Source: CAD feature listing. Evaluate the final solid. Frame: model axes, mm. Face numbers are marked on the shaded views. Give positions to 0.01 mm unless a question says otherwise; leave off trailing zeros. Order: outer loops, then holes, each group sorted by start corner. A loop starts at its lowest first (then second) coordinate and runs counter-clockwise, first axis right, second up.
```python
from build123d import *

# Parameters (mm, degrees)
SKETCH002_W            = 65
SKETCH002_H            = 110
SKETCH002_W_2          = 61
SKETCH002_H_2          = 106
PAD002_DEPTH           = 5
SKETCH003_W            = 65
SKETCH003_H            = 110
SKETCH003_W_2          = 23.5
SKETCH003_H_2          = 98.676263
SKETCH003_H_3          = 24.954477
SKETCH003_H_4          = 22.149553
SKETCH003_H_5          = 22.384941
SKETCH003_H_6          = 10.511029
PAD003_DEPTH           = 2
PAD001_DEPTH           = 10
SKETCH_W               = 59
SKETCH_H               = 10
PAD_DEPTH              = 2
FUSION_PLACEMENT_ANGLE = -33.7
FILLET_R               = 1
FILLET001_R            = 4
FILLET002_R            = 4
FILLET003_R            = 2


with BuildPart() as pad002:
    # Sketch002 → Pad002 (new body)
    with BuildSketch(Plane.XY):
        with Locations((32.5, -56.5)):
            Rectangle(SKETCH002_W, SKETCH002_H)
        with Locations((32.5, -56.5)):
            Rectangle(SKETCH002_W_2, SKETCH002_H_2, mode=Mode.SUBTRACT)
    extrude(amount=PAD002_DEPTH)


with BuildPart() as fusion001:
    # Sketch003 → Pad003 (new body)
    with BuildSketch(Plane.XY):
        with Locations((32.5, -56.5)):
            Rectangle(SKETCH003_W, SKETCH003_H)
        with Locations((17.75, -56.838131)):
            Rectangle(SKETCH003_W_2, SKETCH003_H_2, mode=Mode.SUBTRACT)
        with Locations((47.25, -19.977238)):
            Rectangle(SKETCH003_W_2, SKETCH003_H_3, mode=Mode.SUBTRACT)
        with Locations((47.25, -49.529253)):
            Rectangle(SKETCH003_W_2, SKETCH003_H_4, mode=Mode.SUBTRACT)
        with Locations((47.25, -77.7965)):
            Rectangle(SKETCH003_W_2, SKETCH003_H_5, mode=Mode.SUBTRACT)
        with Locations((47.25, -100.244485)):
            Rectangle(SKETCH003_W_2, SKETCH003_H_6, mode=Mode.SUBTRACT)
    extrude(amount=PAD003_DEPTH)

    # Fusion001: union Pad002
    add(pad002.part)


with BuildPart() as pad001:
    # Sketch001 → Pad001 (new body)
    with BuildSketch(Plane.XY):
        Polygon((0, 0), (0, -8.6), (2.6, -8.6), (2.6, -7.5), (1.1, -7.5), (1.1, -5.5), (2.6, -5.5), (2.6, -1.5), (56.4, -1.5), (56.4, -5.5), (57.9, -5.5), (57.9, -7.5), (56.4, -7.5), (56.4, -8.6), (59, -8.6), (59, 0), align=None)
    extrude(amount=PAD001_DEPTH)


with BuildPart() as relay001:
    # Sketch → Pad (new body)
    with BuildSketch(Plane.XY):
        with Locations((29.5, -5)):
            Rectangle(SKETCH_W, SKETCH_H)
    extrude(amount=PAD_DEPTH)

    # Fusion: union Pad001
    add(pad001.part)


with BuildPart() as relay001_1:
    # Fusion placement: moved
    add(relay001.part.moved(Location((5.548444, -1.680459, 0))).rotate(Axis((5.548444, -1.680459, 0), (0, 0, 1)), FUSION_PLACEMENT_ANGLE))


with BuildPart() as clone_of_relay002:
    # Clone001 base: copy of Relay001
    add(relay001_1.part)


with BuildPart() as clone_of_relay002_1:
    # Clone001 placement: moved
    add(clone_of_relay002.part.moved(Location((0, -56, 0))))


with BuildPart() as fillet003:
    # Clone base: copy of Relay001
    add(relay001_1.part)


with BuildPart() as fillet003_1:
    # Clone placement: moved
    add(fillet003.part.moved(Location((0, -28, 0))))

    # Fusion002: union Fusion001, Clone of Relay002, Relay001
    add(fusion001.part)
    add(clone_of_relay002_1.part)
    add(relay001_1.part)

    # Fillet
    fillet_edges = [fillet003_1.edges().sort_by_distance(p)[0] for p in [
        (49.085293, -98.735821, 1),
        (49.085293, -70.735821, 1),
        (49.085293, -42.735821, 1),
    ]]
    fillet(fillet_edges, radius=FILLET_R)

    # Fillet001
    fillet001_edges = [fillet003_1.edges().sort_by_distance(p)[0] for p in [
        (35.5, -94.988971, 1),
        (43.467128, -94.988971, 1),
        (51.584132, -94.988971, 1),
        (35.5, -66.60403, 1),
        (42.889933, -66.60403, 1),
        (51.840855, -66.60403, 1),
        (35.5, -38.454477, 1),
        (42.665688, -38.454477, 1),
        (51.940595, -38.454477, 1),
        (35.5, -7.5, 1),
        (35.5, -21.655663, 1),
        (51.692138, -32.454477, 1),
        (35.5, -49.655663, 1),
        (51.916383, -60.60403, 1),
        (35.5, -77.655663, 1),
        (52.493578, -88.988971, 1),
        (35.5, -105.5, 1),
        (59, -66.60403, 1),
        (59, -38.454477, 1),
        (59, -7.5, 1),
        (59, -94.988971, 1),
        (59, -105.5, 1),
        (59, -88.988971, 1),
        (59, -60.60403, 1),
        (59, -32.454477, 1),
    ]]
    fillet(fillet001_edges, radius=FILLET001_R)

    # Fillet002
    fillet002_edges = [fillet003_1.edges().sort_by_distance(p)[0] for p in [
        (29.5, -85.674054, 1),
        (29.5, -57.674054, 1),
        (29.5, -29.674054, 1),
        (6, -70.001503, 1),
        (6, -42.001503, 1),
        (6, -14.001503, 1),
        (6, -29.981609, 1),
        (6, -57.981609, 1),
        (6, -106.176263, 1),
        (29.5, -45.654161, 1),
        (29.5, -73.654161, 1),
        (29.5, -106.176263, 1),
    ]]
    fillet(fillet002_edges, radius=FILLET002_R)

    # Fillet003
    fillet003_edges = [fillet003_1.edges().sort_by_distance(p)[0] for p in [
        (29.5, -7.5, 1),
        (14.274478, -7.5, 1),
        (29.5, -17.654161, 1),
    ]]
    fillet(fillet003_edges, radius=FILLET003_R)


solid = fillet003_1.part
```
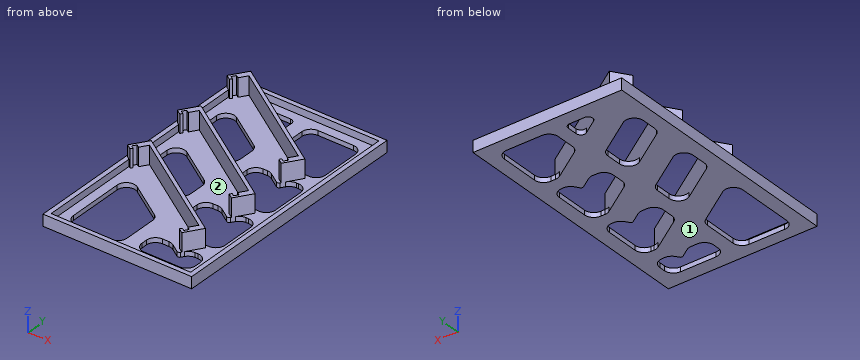
1) Draft query along X for the marked faces 1 and 2. Return one class per face: +X half, -X half, draft (parallel to the pull), parting line (faces both ways), or undercut.
Report:
face 1: draft
face 2: undercut
2) Section query C-C, the plane y = -26. Return the cut outline in (x, z).
Report:
outline: (0, 0) - (6, 0) - (6, 2) - (2, 2) - (2, 5) - (0, 5) - close; (23.99, 0) - (42.01, 0) - (42.01, 10) - (39.31, 10) - (39.31, 2) - (23.99, 2) - close; (59, 0) - (65, 0) - (65, 5) - (63, 5) - (63, 2) - (59, 2) - close
3) Section query B-B, the plane x = 15.5. Return the cut outline in (y, z).
Report:
outline: (-111.5, 0) - (-106.18, 0) - (-106.18, 2) - (-109.5, 2) - (-109.5, 5) - (-111.5, 5) - close; (-76.34, 0) - (-64.32, 0) - (-64.32, 10) - (-66.12, 10) - (-66.12, 2) - (-76.34, 2) - close; (-48.34, 0) - (-36.32, 0) - (-36.32, 10) - (-38.12, 10) - (-38.12, 2) - (-48.34, 2) - close; (-20.34, 0) - (-1.5, 0) - (-1.5, 5) - (-3.5, 5) - (-3.5, 2) - (-8.32, 2) - (-8.32, 10) - (-10.12, 10) - (-10.12, 2) - (-20.34, 2) - close
4) Section query D-D, the plane x = 33. Return the cut outline in (y, z), and give its area (3 significant figures).
Report:
outline: (-111.5, 0) - (-1.5, 0) - (-1.5, 5) - (-3.5, 5) - (-3.5, 2) - (-19.99, 2) - (-19.99, 10) - (-21.79, 10) - (-21.79, 2) - (-47.99, 2) - (-47.99, 10) - (-49.79, 10) - (-49.79, 2) - (-75.99, 2) - (-75.99, 10) - (-77.79, 10) - (-77.79, 2) - (-109.5, 2) - (-109.5, 5) - (-111.5, 5) - close
area: 275 mm2
5) Material intervals for L1, parallel to Y at x = 60, z = 4.75; L2, parallel to Y at x = 39.5, z = 9.25; L3, parallel to Y at x = 54, z = 9, sorted ascending.
Report:
L1: y = -111.5 to -109.5, -3.5 to -1.5
L2: y = -82.13 to -80.32, -54.13 to -52.32, -26.13 to -24.32
L3: y = -91.37 to -89.99, -63.37 to -61.99, -35.37 to -33.99
6) Section query A-A, the plane z = 8.5. Count the separate pieces of the cut face and the enclosed holes in it, and give its area (3 significant figures).
Report:
separate pieces: 3
enclosed holes: 0
area: 358 mm2
7) Pin query (flat end, axial travel): pin 1 (10 mm diameter, centred on x = 12.5, y = -15.5, fed in from +Z). Return the tip coordinate at first contact, or that it passes through.
Report:
pin 1: stops at z = 2
